Source: CAD feature listing. Evaluate the final solid. Frame: model axes, mm. A direction names the side the tool comes from. Round coordinates to 2 decimals unless told otherwise and drop trailing zeros. Answer as CSV lines item,"result". Start each with the question number.
(1) Line query: line 1 along Y through (x, z) = (-11.75, 0); line 2 along Z through (x, y) = (-13, 44); line 3 along Z through (x, y) = (-16, 13). Output: solid intervals per line, ascending. Write a range as from..to.
(2) Set-up query: faces 1 (the flat face through (-13, 50.8, 0)), 2 (the conical face through (2.38, 25.48, -0.05)), 3 (the cylindrical face through (-11.157, 19.374, -1.159)). Return all of +Z, -Z, +X, -X, +Y, -Y with unobstructed straight access to the full face (end or side cutting, diameter ignored); none if empty.
(3) Contact query for flat-ended pins moving along their axis: P1, Ø1.5, axis at x = -12.5, y = 30.5, coming from the +Z side; P2, Ø1, axis at y = 20.5, z = -0.5, coming from the +X side; P3, Ø3, axis at x = -2, z = -1.5, coming from the -Y side; P4, Ø2, axis at x = 0, z = 0, coming from the -Y side. Output: stop coordinate, or through.
(4) Pull-direction query (Y, two-part tool) for faces 4 (the flat face through (-16, 0, 0)), 5 (the flat face through (-14.288, 21, 0)), 6 (the cylindrical face through (-1.713, 6.629, -0.075)); classes: +Y half, -Y half, draft (parallel to the pull), parting line (faces both ways), or undercut.
Autodesk Inventor part; units mm, degrees
ref_plane "Work Plane1" through (0, 50.8, 0) normal (0, 1, 0) x (-1, 0, 0)
ref_plane "YZ Plane" through (0, 0, 0) normal (1, 0, 0) x (0, 1, 0)
ref_plane "XY Plane" through (0, 0, 0) normal (0, 0, 1) x (1, 0, 0)
sketch "Sketch2" plane through (0, 0, 0) normal (0, 1, 0) x (-1, 0, 0)
  circle A0 centre (0, 0) radius 3.175
  line L0 (0, 0) -> (35.56, 0)
  line L1 (0, 3.175) -> (12.2611, 3.175)
  line L2 (0, -3.175) -> (12.3047, -3.175)
  line L3 (13.1799, -3.1144) -> (35.56, 0)
  line L4 (35.56, 0) -> (13.1347, 3.1146)
  arc A1 (13.1347, 3.1146) -> (12.2611, 3.175) centre (12.2611, -3.175) ccw
  arc A2 (12.3047, -3.175) -> (13.1799, -3.1144) centre (12.3047, 3.175) ccw
  circle A3 centre (0, 0) radius 1.5875
  point P0 (12.7, 3.175)
  dimension "d5" = 6.35
  dimension "d6" = 35.56
  dimension "d7" = 12.7
  dimension "d8" = 6.35
  dimension "d9" = 6.35
  dimension "d12" = 3.175
ref_plane "Work Plane1" through (0, 50.8, 0) normal (0, 1, 0) x (-1, 0, 0)
sketch "Sketch3" plane through (0, 50.8, 0) normal (0, 1, 0) x (-1, 0, 0)
  circle A0 centre (0, 0) radius 1.5875
  line L0 (0, 1.5875) -> (12.4798, 1.5875)
  line L1 (0, -1.5875) -> (12.5018, -1.5875)
  line L2 (12.9421, -1.5722) -> (35.56, 0)
  line L3 (35.56, 0) -> (12.9197, 1.5722)
  arc A1 (12.9197, 1.5722) -> (12.4798, 1.5875) centre (12.4798, -4.7625) ccw
  arc A2 (12.5018, -1.5875) -> (12.9421, -1.5722) centre (12.5018, 4.7625) ccw
  point P0 (12.7, 1.5875)
  dimension "d14" = 3.175
  dimension "d15" = 12.7
  dimension "d16" = 6.35
  dimension "d17" = 6.35
loft "Loft1" add profiles "Sketch2", "Sketch3" contours A0 | L0 L3 A2 L2 A0 | A0 L1 A1 L4 L0 | A3 / all
sketch "Sketch4" plane through (0, 0, 0) normal (0, 0, 1) x (1, 0, 0)
  line L0 (-12.2611, 0) -> (0, 0)
  line L1 (0, 0) -> (0, 12.7)
  line L2 (0, 0) -> (0, 50.8)
  line L3 (0, 12.7) -> (-7.9375, 12.7)
  line L4 (-7.9375, 12.7) -> (-7.9375, 20.6375)
  arc A0 (0, 12.7) -> (-7.9375, 20.6375) centre (-7.9375, 12.7) ccw
  line L5 (-7.9375, 20.6375) -> (-14.2875, 20.6375)
  dimension "d22" = 12.7
  dimension "d23" = 7.9375
  dimension "d24" = 7.9375
  dimension "d25" = 6.35
sketch "Sketch5" plane through (-12.3047, 0, -3.175) normal (0, -1, 0) x (1, 0, 0)
  circle A0 centre (12.3047, 3.175) radius 1.7145
  dimension "d26" = 3.429
sweep "Sweep1" cut profiles "Sketch5" path "Sketch4" path curves L1 A0 L5
sketch "Sketch6" plane through (0, 0, 0) normal (0, 0, 1) x (1, 0, 0)
  line L0 (3.175, 0) -> (0, 0)
  line L1 (3.175, 0) -> (-3.175, 0)
  line L2 (0, 0) -> (-12.3047, 0)
  line L3 (-3.175, 0) -> (3.1223, 1.6873)
  line L4 (3.175, 0) -> (1.5875, 50.8)
  dimension "d29" = 6.35
  dimension "d30" = 15
extrude "Extrusion3" cut sketch "Sketch6" along normal mid plane 25.4
properties part number "DivePlanesControlSurface"
Answer block:
1,line 1,"0..18.92, 22.35..50.8"
1,line 2,"-1.78..1.77"
1,line 3,"-2.37..2.37"
2,face 1,"+Z, -Z, +X, -X, +Y"
2,face 2,"+X, +Y"
2,face 3,"none"
3,P1,"z = 2.25"
3,P2,"x = 2.54"
3,P3,"y = 0"
3,P4,"y = 16.34"
4,face 4,"-Y half"
4,face 5,"undercut"
4,face 6,"draft"
